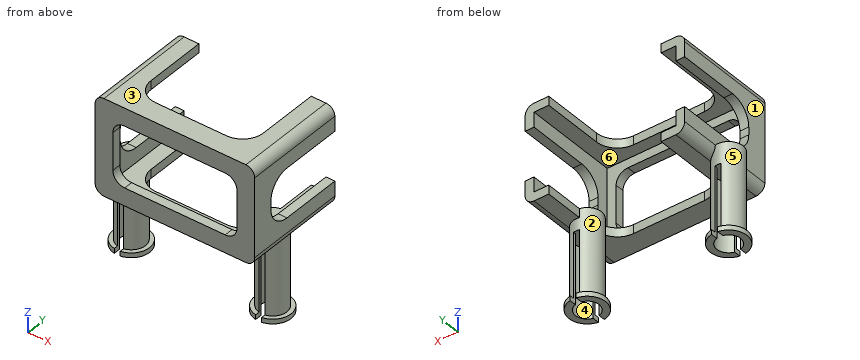
from build123d import *

# Parameters (mm, degrees)
SKETCH1_W                = 27
SKETCH1_H                = 16.3
BOSS_EXTRUDE1_DEPTH      = 17.4
SKETCH2_W                = 24
SKETCH2_H                = 13.3
CUT_EXTRUDE1_DEPTH       = 15.9
SKETCH3_W                = 19
SKETCH3_H                = 16.3
CUT_EXTRUDE2_DEPTH       = 13.9
SKETCH4_W                = 27
SKETCH4_H                = 8.3
CUT_EXTRUDE3_DEPTH       = 13.9
SKETCH6_R                = 3.69
BOSS_EXTRUDE2_DEPTH      = 2.38
SKETCH7_R                = 3.1
CUT_EXTRUDE4_DEPTH       = 0.8
SKETCH8_R                = 2.4
CUT_EXTRUDE5_DEPTH       = 4.8
CUT_EXTRUDE7_START       = -0.8
SKETCH9_R                = 3.1
CUT_EXTRUDE7_DEPTH       = 0.8
CUT_EXTRUDE8_DEPTH       = 10
FILLET1_R                = 3.5
FILLET2_R                = 3.5
FILLET3_R                = 3.5
FILLET4_R                = 3.5
FILLET5_R                = 3.5
FILLET6_R                = 3.5
FILLET7_R                = 3.5
FILLET8_R                = 3.5
FILLET9_R                = 1.5
FILLET10_R               = 1.5
FILLET11_R               = 1.5
FILLET12_R               = 1.5
SKETCH11_W               = 20
SKETCH11_H               = 4.569127273
CUT_EXTRUDE10_DEPTH      = 35
SKETCH12_W               = 26.121320344
SKETCH12_H               = 15.421320343
BOSS_EXTRUDE3_DEPTH      = 1.5
BOSS_EXTRUDE4_DEPTH      = 13.76
BOSS_EXTRUDE4_DEPTH_BACK = 1.5
SKETCH14_R               = 2.4
SKETCH15_R               = 3.1
BOSS_EXTRUDE6_DEPTH      = 0.8
SKETCH17_R               = 2
CUT_EXTRUDE11_DEPTH      = 11.8
SKETCH18_W               = 1
SKETCH18_H               = 8
CUT_EXTRUDE12_DEPTH      = 11.8
BOSS_EXTRUDE7_DEPTH      = 13.803772877
BOSS_EXTRUDE7_DEPTH_BACK = 1.5
SKETCH19_R               = 2.4
SKETCH20_R               = 3.1
BOSS_EXTRUDE8_DEPTH      = 0.8
SKETCH21_R               = 2
CUT_EXTRUDE13_DEPTH      = 11.8
SKETCH22_W               = 1
SKETCH22_H               = 7.748272369
CUT_EXTRUDE14_DEPTH      = 11.8
CUT_EXTRUDE15_DEPTH      = 11.8


with BuildPart() as part:
    # Sketch1 → Boss-Extrude1 (new body)
    with BuildSketch(Plane(origin=(0, 0, 0), x_dir=(1, 0, 0), z_dir=(0, 1, 0))):
        with Locations((-24.874612789, -13.014611924)):
            Rectangle(SKETCH1_W, SKETCH1_H)
    extrude(amount=BOSS_EXTRUDE1_DEPTH)

    # Sketch2 → Cut-Extrude1 (cut)
    with BuildSketch(Plane(origin=(0, 17.4, 0), x_dir=(1, 0, 0), z_dir=(0, 1, 0))):
        with Locations((-24.874612789, -13.014611924)):
            Rectangle(SKETCH2_W, SKETCH2_H)
    extrude(amount=-CUT_EXTRUDE1_DEPTH, mode=Mode.SUBTRACT)

    # Sketch3 → Cut-Extrude2 (cut)
    with BuildSketch(Plane(origin=(0, 17.4, 0), x_dir=(1, 0, 0), z_dir=(0, 1, 0))):
        with Locations((-24.874612789, -13.014611924)):
            Rectangle(SKETCH3_W, SKETCH3_H)
    extrude(amount=-CUT_EXTRUDE2_DEPTH, mode=Mode.SUBTRACT)

    # Sketch4 → Cut-Extrude3 (cut)
    with BuildSketch(Plane(origin=(0, 17.4, 0), x_dir=(1, 0, 0), z_dir=(0, 1, 0))):
        with Locations((-24.874612789, -13.014611924)):
            Rectangle(SKETCH4_W, SKETCH4_H)
    extrude(amount=-CUT_EXTRUDE3_DEPTH, mode=Mode.SUBTRACT)

    # Sketch6 → Boss-Extrude2 (add)
    with BuildSketch(Plane(origin=(0, 0, 0), x_dir=(-1, 0, 0), z_dir=(0, -1, 0))):
        with Locations(Location((32.844612789, -9.029611924, 0), (0, 0, 90))):
            Circle(SKETCH6_R)
        with Locations(Location((32.844612789, -16.999611924, 0), (0, 0, 90))):
            Circle(SKETCH6_R)
        with Locations(Location((16.904612789, -9.029611924, 0), (0, 0, 90))):
            Circle(SKETCH6_R)
        with Locations(Location((16.904612789, -16.999611924, 0), (0, 0, 90))):
            Circle(SKETCH6_R)
    extrude(amount=BOSS_EXTRUDE2_DEPTH)

    # Sketch7 → Cut-Extrude4 (cut)
    with BuildSketch(Plane(origin=(0, -2.38, 0), x_dir=(-1, 0, 0), z_dir=(0, -1, 0))):
        with Locations(Location((32.844612789, -9.029611924, 0), (0, 0, 90))):
            Circle(SKETCH7_R)
        with Locations(Location((32.844612789, -16.999611924, 0), (0, 0, 90))):
            Circle(SKETCH7_R)
        with Locations(Location((16.904612789, -16.999611924, 0), (0, 0, 90))):
            Circle(SKETCH7_R)
        with Locations(Location((16.904612789, -9.029611924, 0), (0, 0, 90))):
            Circle(SKETCH7_R)
    extrude(amount=-CUT_EXTRUDE4_DEPTH, mode=Mode.SUBTRACT)

    # Sketch8 → Cut-Extrude5 (cut)
    with BuildSketch(Plane(origin=(0, -1.58, 0), x_dir=(-1, 0, 0), z_dir=(0, -1, 0))):
        with Locations(Location((32.844612789, -9.029611924, 0), (0, 0, 90))):
            Circle(SKETCH8_R)
        with Locations(Location((32.844612789, -16.999611924, 0), (0, 0, 90))):
            Circle(SKETCH8_R)
        with Locations(Location((16.904612789, -16.999611924, 0), (0, 0, 90))):
            Circle(SKETCH8_R)
        with Locations(Location((16.904612789, -9.029611924, 0), (0, 0, 90))):
            Circle(SKETCH8_R)
    extrude(amount=-CUT_EXTRUDE5_DEPTH, mode=Mode.SUBTRACT)

    # Sketch9 → Cut-Extrude7 (cut)
    with BuildSketch(Plane(origin=(0, 1.5, 0), x_dir=(1, 0, 0), z_dir=(0, 1, 0)).offset(CUT_EXTRUDE7_START)):
        with Locations(Location((-16.904612789, -16.999611924, 0), (0, 0, 90))):
            Circle(SKETCH9_R)
        with Locations(Location((-16.904612789, -9.029611924, 0), (0, 0, 90))):
            Circle(SKETCH9_R)
        with Locations(Location((-32.844612789, -9.029611924, 0), (0, 0, 90))):
            Circle(SKETCH9_R)
        with Locations(Location((-32.844612789, -16.999611924, 0), (0, 0, 90))):
            Circle(SKETCH9_R)
    extrude(amount=CUT_EXTRUDE7_DEPTH, mode=Mode.SUBTRACT)

    # Sketch10 → Cut-Extrude8 (cut)
    with BuildSketch(Plane(origin=(0, 1.5, 0), x_dir=(1, 0, 0), z_dir=(0, 1, 0))):
        with BuildLine():
            Line((-22.404612789, -7.864611924), (-27.344612789, -7.864611924))
            ThreePointArc((-27.344612789, -7.864611924), (-28.405272961, -8.303951753), (-28.844612789, -9.364611924))
            Line((-28.844612789, -9.364611924), (-28.844612789, -16.664611924))
            ThreePointArc((-28.844612789, -16.664611924), (-28.405272961, -17.725272096), (-27.344612789, -18.164611924))
            Line((-27.344612789, -18.164611924), (-22.404612789, -18.164611924))
            ThreePointArc((-22.404612789, -18.164611924), (-21.343952617, -17.725272096), (-20.904612789, -16.664611924))
            Line((-20.904612789, -16.664611924), (-20.904612789, -9.364611924))
            ThreePointArc((-20.904612789, -9.364611924), (-21.343952617, -8.303951753), (-22.404612789, -7.864611924))
        make_face()
    extrude(amount=-CUT_EXTRUDE8_DEPTH, mode=Mode.SUBTRACT)

    # Fillet1
    fillet1_edges = [part.edges().sort_by_distance(p)[0] for p in [
        (-15.374612789, 3.5, 5.614611924),
    ]]
    fillet(fillet1_edges, radius=FILLET1_R)

    # Fillet2
    fillet2_edges = [part.edges().sort_by_distance(p)[0] for p in [
        (-15.374612789, 3.5, 20.414611924),
    ]]
    fillet(fillet2_edges, radius=FILLET2_R)

    # Fillet3
    fillet3_edges = [part.edges().sort_by_distance(p)[0] for p in [
        (-12.124612789, 3.5, 17.164611924),
    ]]
    fillet(fillet3_edges, radius=FILLET3_R)

    # Fillet4
    fillet4_edges = [part.edges().sort_by_distance(p)[0] for p in [
        (-12.124612789, 3.5, 8.864611924),
    ]]
    fillet(fillet4_edges, radius=FILLET4_R)

    # Fillet5
    fillet5_edges = [part.edges().sort_by_distance(p)[0] for p in [
        (-37.624612789, 3.5, 8.864611924),
    ]]
    fillet(fillet5_edges, radius=FILLET5_R)

    # Fillet6
    fillet6_edges = [part.edges().sort_by_distance(p)[0] for p in [
        (-37.624612789, 3.5, 17.164611924),
    ]]
    fillet(fillet6_edges, radius=FILLET6_R)

    # Fillet7
    fillet7_edges = [part.edges().sort_by_distance(p)[0] for p in [
        (-34.374612789, 3.5, 5.614611924),
    ]]
    fillet(fillet7_edges, radius=FILLET7_R)

    # Fillet8
    fillet8_edges = [part.edges().sort_by_distance(p)[0] for p in [
        (-34.374612789, 3.5, 20.414611924),
    ]]
    fillet(fillet8_edges, radius=FILLET8_R)

    # Fillet9
    fillet9_edges = [part.edges().sort_by_distance(p)[0] for p in [
        (-38.374612789, 8.7, 21.164611924),
    ]]
    fillet(fillet9_edges, radius=FILLET9_R)

    # Fillet10
    fillet10_edges = [part.edges().sort_by_distance(p)[0] for p in [
        (-38.374612789, 8.7, 4.864611924),
    ]]
    fillet(fillet10_edges, radius=FILLET10_R)

    # Fillet11
    fillet11_edges = [part.edges().sort_by_distance(p)[0] for p in [
        (-11.374612789, 8.7, 4.864611924),
    ]]
    fillet(fillet11_edges, radius=FILLET11_R)

    # Fillet12
    fillet12_edges = [part.edges().sort_by_distance(p)[0] for p in [
        (-11.374612789, 8.7, 21.164611924),
    ]]
    fillet(fillet12_edges, radius=FILLET12_R)

    # Sketch11 → Cut-Extrude10 (cut)
    with BuildSketch(Plane(origin=(-11.374612789, 0, 0), x_dir=(0, 0, -1), z_dir=(1, 0, 0))):
        with Locations((-11.164611924, -2.284563637)):
            Rectangle(SKETCH11_W, SKETCH11_H)
    extrude(amount=-CUT_EXTRUDE10_DEPTH, mode=Mode.SUBTRACT)

    # Sketch12 → Boss-Extrude3 (add)
    with BuildSketch(Plane(origin=(0, 0, 0), x_dir=(-1, 0, 0), z_dir=(0, -1, 0))):
        with Locations((24.874612789, -13.014611925)):
            Rectangle(SKETCH12_W, SKETCH12_H)
    extrude(amount=-BOSS_EXTRUDE3_DEPTH)

    # Sketch14 → Boss-Extrude4 (add, two sides: drawn at the far end of the back side and taken through both)
    with BuildSketch(Plane(origin=(-4.421362725, 0, 4.864611924), x_dir=(-1, 0, 0), z_dir=(0, 0, -1)).offset(-BOSS_EXTRUDE4_DEPTH_BACK)):
        with Locations(Location((34.374612789, 8.4, 0), (0, 0, 143.184357726))):
            Circle(SKETCH14_R)
    extrude(amount=BOSS_EXTRUDE4_DEPTH + BOSS_EXTRUDE4_DEPTH_BACK)

    # Sketch15 → Boss-Extrude6 (add)
    with BuildSketch(Plane(origin=(-4.421362725, 0, -8.895388076), x_dir=(-1, 0, 0), z_dir=(0, 0, -1))):
        with Locations((34.374612789, 8.4)):
            Circle(SKETCH15_R)
    extrude(amount=-BOSS_EXTRUDE6_DEPTH)

    # Sketch17 → Cut-Extrude11 (cut)
    with BuildSketch(Plane(origin=(-4.421362725, 0, -8.895388076), x_dir=(-1, 0, 0), z_dir=(0, 0, -1))):
        with Locations((34.374612789, 8.4)):
            Circle(SKETCH17_R)
    extrude(amount=-CUT_EXTRUDE11_DEPTH, mode=Mode.SUBTRACT)

    # Sketch18 → Cut-Extrude12 (cut)
    with BuildSketch(Plane(origin=(-4.421362725, 0, -8.895388076), x_dir=(-1, 0, 0), z_dir=(0, 0, -1))):
        with Locations((34.374612789, 8.4)):
            Rectangle(SKETCH18_W, SKETCH18_H)
    extrude(amount=-CUT_EXTRUDE12_DEPTH, mode=Mode.SUBTRACT)

    # Sketch19 → Boss-Extrude7 (add, two sides: drawn at the far end of the back side and taken through both)
    with BuildSketch(Plane(origin=(0, 0, 4.864611924), x_dir=(-1, 0, 0), z_dir=(0, 0, -1)).offset(-BOSS_EXTRUDE7_DEPTH_BACK)):
        with Locations((14.875975514, 8.4)):
            Circle(SKETCH19_R)
    extrude(amount=BOSS_EXTRUDE7_DEPTH + BOSS_EXTRUDE7_DEPTH_BACK)

    # Sketch20 → Boss-Extrude8 (add)
    with BuildSketch(Plane(origin=(0, 0, -8.939160952), x_dir=(-1, 0, 0), z_dir=(0, 0, -1))):
        with Locations((14.875975514, 8.4)):
            Circle(SKETCH20_R)
    extrude(amount=-BOSS_EXTRUDE8_DEPTH)

    # Sketch21 → Cut-Extrude13 (cut)
    with BuildSketch(Plane(origin=(0, 0, -8.939160952), x_dir=(-1, 0, 0), z_dir=(0, 0, -1))):
        with Locations((14.875975514, 8.4)):
            Circle(SKETCH21_R)
    extrude(amount=-CUT_EXTRUDE13_DEPTH, mode=Mode.SUBTRACT)

    # Sketch22 → Cut-Extrude14 (cut)
    with BuildSketch(Plane(origin=(0, 0, -8.939160952), x_dir=(-1, 0, 0), z_dir=(0, 0, -1))):
        with Locations((14.875975514, 8.525863815)):
            Rectangle(SKETCH22_W, SKETCH22_H)
    extrude(amount=-CUT_EXTRUDE14_DEPTH, mode=Mode.SUBTRACT)

    # Sketch23 → Cut-Extrude15 (cut)
    with BuildSketch(Plane(origin=(0, 1.5, 0), x_dir=(1, 0, 0), z_dir=(0, 1, 0))):
        with BuildLine():
            Line((-33.374612789, -7.864611924), (-16.374612789, -7.864611924))
            ThreePointArc((-16.374612789, -7.864611924), (-14.960399227, -8.450398362), (-14.374612789, -9.864611924))
            Line((-14.374612789, -9.864611924), (-14.374612789, -16.164611924))
            ThreePointArc((-14.374612789, -16.164611924), (-14.960399227, -17.578825487), (-16.374612789, -18.164611924))
            Line((-16.374612789, -18.164611924), (-33.374612789, -18.164611924))
            ThreePointArc((-33.374612789, -18.164611924), (-34.788826352, -17.578825487), (-35.374612789, -16.164611924))
            Line((-35.374612789, -16.164611924), (-35.374612789, -9.864611924))
            ThreePointArc((-35.374612789, -9.864611924), (-34.788826352, -8.450398362), (-33.374612789, -7.864611924))
        make_face()
    extrude(amount=-CUT_EXTRUDE15_DEPTH, mode=Mode.SUBTRACT)


solid = part.part
Design review of the part built by this model. Coordinates are the model's own, in mm. Face numbers are marked on the shaded views. A direction names the side the tool comes from. Coordinates: 2 decimals unless noted, no trailing zeros. Write each loop counter-clockwise with the first axis right and the second up, starting at its lowest first coordinate (ties: lowest second). Pieces come first, ordered by that corner, then holes. Notation, with made-up numbers: (-21, 78) -> (-7, 78) arc R15 cw to (-7, 86) -> close; hole circle Ø4 at (14, 70). An arc over 180 degrees is marked (long way). Write each question's results on one line, items separated by ' | '. Start each with the question number.
(1) The part is to be moulded in two halves that separate along Z. For the marked faces 1, 2 and 3, say which applies: pulls with the +Z half, pulls with the -Z half, needs draft (parallel to the pull), parting line crosses it, or undercut.
(2) Take a section at C-C on z = 3.5. Write out the cut boundary in (x, y), and give its area (3 significant figures).
(3) Take a section at A-A on y = 14. Write out the cut boundary in (x, z).
(4) For line 1 along X through (y, z) = (8.25, -3); line 2 along X through (y, z) = (15.5, 6.5); line 3 along Z through (x, y) = (-23.5, 1), list the stretches that pass through material, from the lowest coordinate up. Write a range as from..to.
(5) Tool access review of the marked faces 4, 5 and 6: name each direction out of +Z, -Z, +X, -X, +Y, -Y from which nothing blocks a thin tool from reaching the whole face with its end or side.
(6) Clearance check with flat-ended pins moving along their axes: P1, Ø3, axis at x = -39.5, y = 7.5, coming from the -Z side; P2, Ø1.2, axis at x = -37.5, y = 13, coming from the +Z side; P3, Ø0.9, axis at y = 6, z = -0.5, coming from the +X side; P4, Ø0.6, axis at y = 6, z = -4.5, coming from the -X side. State where each tip first meets the part, or that it passes through.
(7) Take a section at B-B on x = -28. Write out the cut boundary in (y, z), and give its area (3 significant figures).
(8) Take a section at D-D on y = 4. Write out the cut boundary in (x, z), and give its area (3 significant figures).
Results found:
1) face 1: needs draft | face 2: undercut | face 3: pulls with the +Z half
2) outline: circle Ø4.8 at (-38.8, 8.4); circle Ø4.8 at (-14.88, 8.4) | area: 36.2 mm2
3) outline: (-38.37, 6.36) arc R1.5 ccw to (-36.87, 4.86) -> (-34.37, 4.86) -> (-34.37, 6.36) -> (-36.87, 6.36) -> (-36.87, 8.86) -> (-38.37, 8.86) -> close; (-38.37, 17.16) -> (-36.87, 17.16) -> (-36.87, 19.66) -> (-34.37, 19.66) -> (-34.37, 21.16) -> (-36.87, 21.16) arc R1.5 ccw to (-38.37, 19.66) -> close; (-15.37, 4.86) -> (-12.87, 4.86) arc R1.5 ccw to (-11.37, 6.36) -> (-11.37, 8.86) -> (-12.87, 8.86) -> (-12.87, 6.36) -> (-15.37, 6.36) -> close; (-15.37, 19.66) -> (-12.87, 19.66) -> (-12.87, 17.16) -> (-11.37, 17.16) -> (-11.37, 19.66) arc R1.5 ccw to (-12.87, 21.16) -> (-15.37, 21.16) -> close
4) line 1: x = -41.19..-40.79, -36.8..-36.4, -17.27..-16.87, -12.88..-12.48 | line 2: x = -38.37..-36.87, -12.87..-11.37 | line 3: z = 4.86..7.86, 18.16..21.16
5) face 4: -Z | face 5: none | face 6: +Y
6) P1: stops at z = -8.9 | P2: stops at z = 21.16 | P3: stops at x = -13.48 | P4: stops at x = -39.96
7) outline: (0, 4.86) -> (3.5, 4.86) -> (3.5, 6.36) -> (1.5, 6.36) -> (1.5, 7.86) -> (0, 7.86) -> close; (0, 18.16) -> (1.5, 18.16) -> (1.5, 19.66) -> (3.5, 19.66) -> (3.5, 21.16) -> (0, 21.16) -> close | area: 15.0 mm2
8) outline: (-38.37, 6.36) arc R1.5 ccw to (-36.87, 4.86) -> (-32.68, 4.86) -> (-32.68, 6.36) -> (-36.87, 6.36) -> (-36.87, 10.56) -> (-38.37, 10.56) -> close; (-38.37, 15.47) -> (-36.87, 15.47) -> (-36.87, 19.66) -> (-32.68, 19.66) -> (-32.68, 21.16) -> (-36.87, 21.16) arc R1.5 ccw to (-38.37, 19.66) -> close; (-17.07, 4.86) -> (-12.87, 4.86) arc R1.5 ccw to (-11.37, 6.36) -> (-11.37, 10.56) -> (-12.87, 10.56) -> (-12.87, 6.36) -> (-17.07, 6.36) -> close; (-17.07, 19.66) -> (-12.87, 19.66) -> (-12.87, 15.47) -> (-11.37, 15.47) -> (-11.37, 19.66) arc R1.5 ccw to (-12.87, 21.16) -> (-17.07, 21.16) -> close | area: 57.4 mm2
